The model under review builds one solid part; all positions refer to its coordinate system, in mm. Face numbers are marked on the shaded views. A direction names the side the tool comes from. Coordinates: 2 decimals unless noted, no trailing zeros. Write each loop counter-clockwise with the first axis right and the second up, starting at its lowest first coordinate (ties: lowest second). Pieces come first, ordered by that corner, then holes. Notation, with made-up numbers: (-32.75, 5) - (-2.75, 5) arc R26 ccw to (-2.75, 37) - close; hole circle Ø8 at (64.25, 72.25). An arc over 180 degrees is marked (long way). Return JSON: item names as keys, results as strings. Group by question number.
(1) We need section B-B on y = 0. State the section outline as (x, z) points.
(2) We need section D-D on y = 114. State the section outline as (x, z) points.
(3) We need section C-C on z = -13. State the section outline as (x, y) points.
(4) For pin 1 Ø8 at (y, z) = (171, -18.5) entering from -X; pin 2 Ø6 at (x, z) = (-311.5, -69) entering from +Y; pin 3 Ø5 at (x, y) = (31.5, 197) entering from -Z, all flat-tipped, find the tip position at first contact; note any pin that passes through.
(5) We need section A-A on x = 0. State the section outline as (y, z) points, then the cut area to 3 significant figures.
(6) To check wall thickness, follow L1, parallel to X at y = -125, z = -108.5; L2, parallel to Y at x = -122, z = -3; L3, parallel to Y at x = 0, z = 145. State the ranges of each line that lie inside material, in increasing order. Write a range as from..to.
(7) Draft analysis for pull direction X (two halves, no side actions). For the marked faces 1, 2 and 3, state which applies: released by +X, released by -X, zero draft, split by the parting line, or undercut.
(8) Tool access review of the marked faces 4, 5, 6 and 7: name each direction out of +Z, -Z, +X, -X, +Y, -Y from which nothing blocks a thin tool from reaching the whole face with its end or side.
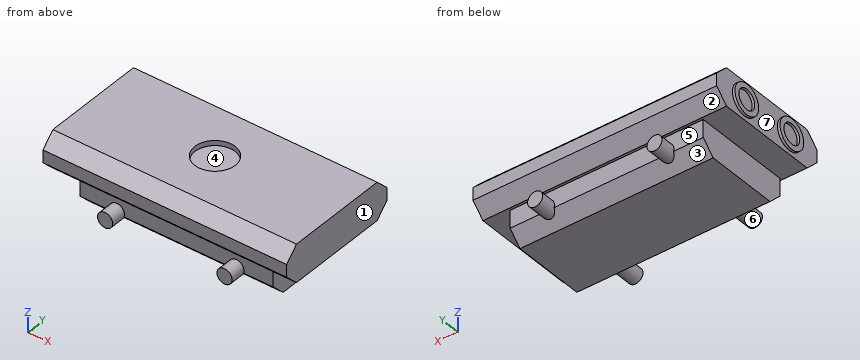
```python
from build123d import *

# Parameters (mm, degrees)
SKETCH1_W            = 965
SKETCH1_H            = 508
BOSS_EXTRUDE1_DEPTH  = 150
SKETCH2_W            = 765
SKETCH2_H            = 388
BOSS_EXTRUDE2_DEPTH  = 120
SKETCH3_R            = 30
BOSS_EXTRUDE3_DEPTH  = 60
LPATTERN2_COUNT      = 2
LPATTERN2_PITCH      = 448
LPATTERN2_COUNT_DIR2 = 2
LPATTERN2_PITCH_DIR2 = 473
CHAMFER1_SIZE        = 50
SKETCH4_R            = 60
SKETCH4_R_2          = 40
BOSS_EXTRUDE4_DEPTH  = 10
SKETCH5_R            = 80
CUT_EXTRUDE1_DEPTH   = 20


with BuildPart() as part:
    # Sketch1 → Boss-Extrude1 (new body)
    with BuildSketch(Plane.XY):
        Rectangle(SKETCH1_W, SKETCH1_H)
    extrude(amount=BOSS_EXTRUDE1_DEPTH)


with BuildPart() as body_2:
    # Sketch2 → Boss-Extrude2 (new body)
    with BuildSketch(Plane.XY):
        Rectangle(SKETCH2_W, SKETCH2_H)
    extrude(amount=-BOSS_EXTRUDE2_DEPTH)


with BuildPart() as body_3:
    # Sketch3 → Boss-Extrude3 (new body)
    with BuildSketch(Plane.XZ.offset(194)):
        with Locations(Location((236.5, -60, 0), (0, 0, 270))):
            Circle(SKETCH3_R)
    boss_extrude3 = extrude(amount=BOSS_EXTRUDE3_DEPTH)


with BuildPart() as lpattern2_1:
    # LPattern2: pattern copy
    add(boss_extrude3.moved(Location(Vector(0, 1, 0) * (0 * LPATTERN2_PITCH) + Vector(-1, 0, 0) * (1 * LPATTERN2_PITCH_DIR2))))


with BuildPart() as lpattern2_2:
    # LPattern2: pattern copy
    add(boss_extrude3.moved(Location(Vector(0, 1, 0) * (1 * LPATTERN2_PITCH) + Vector(-1, 0, 0) * (0 * LPATTERN2_PITCH_DIR2))))


with BuildPart() as lpattern2_3:
    # LPattern2: pattern copy
    add(boss_extrude3.moved(Location(Vector(0, 1, 0) * (1 * LPATTERN2_PITCH) + Vector(-1, 0, 0) * (1 * LPATTERN2_PITCH_DIR2))))


with BuildPart() as part_1:
    add(part.part)

    # Combine1: union body 2
    add(body_2.part)

    # Combine4: union body 3, LPattern2_1
    add(body_3.part)
    add(lpattern2_1.part)


with BuildPart() as lpattern2_2_1:
    add(lpattern2_2.part)

    # Combine5: union LPattern2_3, part
    add(lpattern2_3.part)
    add(part_1.part)

    # Chamfer1
    # the kernel refuses this chamfer: 50 mm, written as the material it takes off along each edge
    with BuildSketch(Plane(origin=(611.084149398, -254, 0), x_dir=(0, -0.027495876610586594, 0.9996219169112966), z_dir=(-1, 0, 0)), Plane(origin=(-611.084149398, 254, 150), x_dir=(0, -0.9996219169112966, 0.027495876610586587), z_dir=(1, 0, 0))) as chamfer1_piece_1:
        Polygon((CHAMFER1_SIZE * 0.999621916911, CHAMFER1_SIZE * 0.0274958766106), (-CHAMFER1_SIZE * 0.0274958766106, CHAMFER1_SIZE * 0.999621916911), (0, 0), align=None)
    extrude(amount=1222.168298797, mode=Mode.SUBTRACT)
    with BuildSketch(Plane(origin=(-611.084149398, 254, 0), x_dir=(0, -0.9996219169112966, -0.02749587661058636), z_dir=(1, 0, 0)), Plane(origin=(611.084149398, -254, 150), x_dir=(0, -0.027495876610586594, -0.9996219169112966), z_dir=(-1, 0, 0))) as chamfer1_piece_2:
        Polygon((CHAMFER1_SIZE * 0.999621916911, -CHAMFER1_SIZE * 0.0274958766106), (-CHAMFER1_SIZE * 0.0274958766106, -CHAMFER1_SIZE * 0.999621916911), (0, 0), align=None)
    extrude(amount=1222.168298797, mode=Mode.SUBTRACT)
    with BuildSketch(Plane(origin=(-511.084149398, 194, -120), x_dir=(0, 0.027495876610586594, 0.9996219169112966), z_dir=(1, 0, 0))) as chamfer1_piece_3_section:
        Polygon((CHAMFER1_SIZE * 0.999621916911, CHAMFER1_SIZE * 0.0274958766106), (-CHAMFER1_SIZE * 0.0274958766106, CHAMFER1_SIZE * 0.999621916911), (0, 0), align=None)
    chamfer1_piece_3 = extrude(amount=1022.168298797, mode=Mode.PRIVATE)
    chamfer1_piece_3 = chamfer1_piece_3 - Plane(origin=(-236.5, 177.365883925, -60), x_dir=(0, 0, -1), z_dir=(0, 1, 0)) * Cylinder(30, 2245, mode=Mode.PRIVATE)
    chamfer1_piece_3 = chamfer1_piece_3 - Plane(origin=(236.5, 177.365883925, -60), x_dir=(0, 0, -1), z_dir=(0, 1, 0)) * Cylinder(30, 2245, mode=Mode.PRIVATE)
    add(chamfer1_piece_3, mode=Mode.SUBTRACT)
    with BuildSketch(Plane(origin=(511.084149398, -194, -120), x_dir=(0, -0.027495876610586594, 0.9996219169112966), z_dir=(-1, 0, 0))) as chamfer1_piece_4_section:
        Polygon((CHAMFER1_SIZE * 0.999621916911, CHAMFER1_SIZE * 0.0274958766106), (-CHAMFER1_SIZE * 0.0274958766106, CHAMFER1_SIZE * 0.999621916911), (0, 0), align=None)
    chamfer1_piece_4 = extrude(amount=1022.168298797, mode=Mode.PRIVATE)
    chamfer1_piece_4 = chamfer1_piece_4 - Plane(origin=(236.5, -177.365883925, -60), x_dir=(0, 0, -1), z_dir=(0, 1, 0)) * Cylinder(30, 2245, mode=Mode.PRIVATE)
    chamfer1_piece_4 = chamfer1_piece_4 - Plane(origin=(-236.5, -177.365883925, -60), x_dir=(0, 0, -1), z_dir=(0, 1, 0)) * Cylinder(30, 2245, mode=Mode.PRIVATE)
    add(chamfer1_piece_4, mode=Mode.SUBTRACT)

    # Sketch4 → Boss-Extrude4 (add)
    # profile 1 of 2: a face of its own
    with BuildSketch(Plane.ZY.offset(482.5)):
        with Locations(Location((75, 114, 0), (0, 0, 180))):
            Circle(SKETCH4_R)
        with Locations((75, 114)):
            Circle(SKETCH4_R_2, mode=Mode.SUBTRACT)
    # profile 2 of 2: a face of its own
    with BuildSketch(Plane.ZY.offset(482.5)):
        with Locations(Location((75, -114, 0), (0, 0, 180))):
            Circle(SKETCH4_R)
        with Locations((75, -114)):
            Circle(SKETCH4_R_2, mode=Mode.SUBTRACT)
    extrude(amount=BOSS_EXTRUDE4_DEPTH)

    # Sketch5 → Cut-Extrude1 (cut)
    with BuildSketch(Plane.XY.offset(150)):
        Circle(SKETCH5_R)
    extrude(amount=-CUT_EXTRUDE1_DEPTH, mode=Mode.SUBTRACT)


solid = lpattern2_2_1.part
```
Ans:
{
 "1": {"outline": "(-482.5, 0) - (-382.5, 0) - (-382.5, -120) - (382.5, -120) - (382.5, 0) - (482.5, 0) - (482.5, 150) - (80, 150) - (80, 130) - (-80, 130) - (-80, 150) - (-482.5, 150) - close"},
 "2": {"outline": "(-492.5, 15) - (-482.5, 15) - (-482.5, 0) - (-382.5, 0) - (-382.5, -120) - (382.5, -120) - (382.5, 0) - (482.5, 0) - (482.5, 150) - (-482.5, 150) - (-482.5, 135) - (-492.5, 135) - (-492.5, 115) - (-482.5, 115) - (-482.5, 35) - (-492.5, 35) - close"},
 "3": {"outline": "(-382.5, -194) - (382.5, -194) - (382.5, 194) - (-382.5, 194) - close"},
 "4": {"pin 1": "x = -382.5", "pin 2": "y = 194", "pin 3": "z = 0"},
 "5": {"outline": "(-254, 50) - (-204, 0) - (-194, 0) - (-194, -70) - (-144, -120) - (144, -120) - (194, -70) - (194, 0) - (204, 0) - (254, 50) - (254, 100) - (204, 150) - (80, 150) - (80, 130) - (-80, 130) - (-80, 150) - (-204, 150) - (-254, 100) - close", "area": "112,000 mm²"},
 "6": {"L1": "-382.5..382.5", "L2": "-194..194", "L3": "-209..-80, 80..209"},
 "7": {"face 1": "released by +X", "face 2": "zero draft", "face 3": "undercut"},
 "8": {"face 4": "+Z", "face 5": "+Y", "face 6": "-Y", "face 7": "-X"}
}
